Could you check a few things on this model? Use its own coordinates, in mm. Face numbers are marked on the shaded views. A direction names the side the tool comes from. Give positions to 0.01 mm unless a question says otherwise; leave off trailing zeros. Order: outer loops, then holes, each group sorted by start corner. A loop starts at its lowest first (then second) coordinate and runs counter-clockwise, first axis right, second up. Notation, with made-up numbers: (19, 66.5) - (67, 66.5) arc R31 ccw to (67, 99.5) - close; hole circle Ø1 at (81.5, 74.25). An arc over 180 degrees is marked (long way). One line per question, with ' | ' between items. Start each with the question number.
1. Imagine slicing it at A-A (y = 0). Please give me the cut outline in (x, z), and give its area (3 significant figures).
2. I need wall thicknesses on probe 1 along Y at (x, z) = (0, 1); probe 2 along Z at (x, y) = (7.25, -0.5); probe 3 along Z at (x, y) = (-5.5, -1). Which ranges of each line are inside material? Lowest first, please. Write a range as from..to.
3. For P1, Ø3, axis at y = 5.5, z = 3, coming from the -X side; P2, Ø3, axis at x = -5.5, z = 0, coming from the -Y side, each with a flat end and sliding along its axis, tell me the tip position at first contact or that it passes through.
4. Imagine slicing it at C-C (z = 2.3). Please give me the cut outline in (x, y), and give its area (3 significant figures).
5. Which directions (+Z, -Z, +X, -X, +Y, -Y) give clear straight access to the entire face, cutting with the end or side of a thin tool? Please do the marked faces 4 and 5.
6. If we mould it in two halves opening along X, with no side actions, what happens to the marked faces 1, 2 and 3? For each: released by +X, released by -X, zero draft, split by the parting line, or undercut.
```python
from build123d import *

# Parameters (mm, degrees)
F0_R     = 12
F0_R_2   = 6.5
F0_R_3   = 3.6
F0_R_4   = 1.75
F1_DEPTH = 1.5
F2_DEPTH = 3.5
F3_DEPTH = 0.8
F4_SIZE  = 1


with BuildPart() as f1:
    # F0 (on Top) → F1 (new body)
    with BuildSketch(Plane.XY):
        Circle(F0_R)
        Circle(F0_R_2, mode=Mode.SUBTRACT)
        Circle(F0_R_2)
        Circle(F0_R_3, mode=Mode.SUBTRACT)
        Circle(F0_R_3)
        Circle(F0_R_4, mode=Mode.SUBTRACT)
    extrude(amount=-F1_DEPTH)

    # F0 (on Top) → F2 (join)
    with BuildSketch(Plane.XY):
        Circle(F0_R_3)
        Circle(F0_R_4, mode=Mode.SUBTRACT)
    extrude(amount=F2_DEPTH)

    # F0 (on Top) → F3 (join)
    with BuildSketch(Plane.XY):
        Circle(F0_R_2)
        Circle(F0_R_3, mode=Mode.SUBTRACT)
    extrude(amount=F3_DEPTH)

    # F4
    f4_edges = [f1.edges().sort_by_distance(p)[0] for p in [
        (-12, 0, -1.5),
    ]]
    chamfer(f4_edges, length=F4_SIZE)


solid = f1.part
```
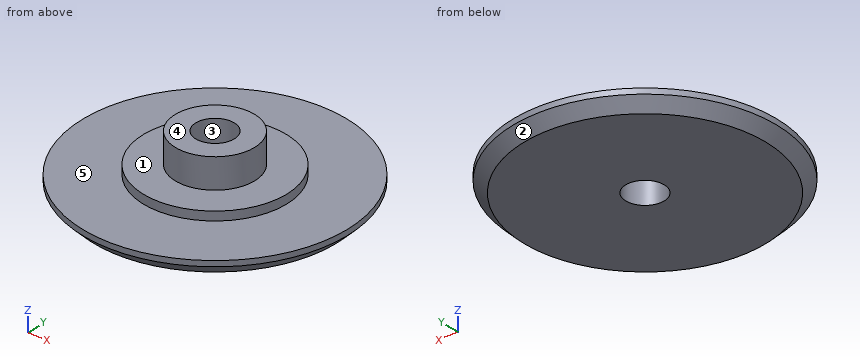
Results found:
1) outline: (-12, -0.5) - (-11, -1.5) - (-1.75, -1.5) - (-1.75, 3.5) - (-3.6, 3.5) - (-3.6, 0.8) - (-6.5, 0.8) - (-6.5, 0) - (-12, 0) - close; (1.75, -1.5) - (11, -1.5) - (12, -0.5) - (12, 0) - (6.5, 0) - (6.5, 0.8) - (3.6, 0.8) - (3.6, 3.5) - (1.75, 3.5) - close | area: 47.3 mm2
2) probe 1: y = -3.6..-1.75, 1.75..3.6 | probe 2: z = -1.5..0 | probe 3: z = -1.5..0.8
3) P1: passes through | P2: stops at y = -11.31
4) outline: circle Ø7.2 at (0, 0); hole circle Ø3.5 at (0, 0) | area: 31.1 mm2
5) face 4: +Z, +X, -X, +Y, -Y | face 5: +Z
6) face 1: zero draft | face 2: split by the parting line | face 3: undercut
